from build123d import *

# Parameters (mm, degrees)
SKETCH3_W           = 80
SKETCH3_H           = 110
BOSS_EXTRUDE1_DEPTH = 6
SKETCH4_W           = 6
SKETCH4_H           = 4
BOSS_EXTRUDE2_DEPTH = 6
SKETCH6_W           = 10
SKETCH6_H           = 5
BOSS_EXTRUDE3_DEPTH = 6
SKETCH8_R           = 12.4841
CUT_EXTRUDE1_DEPTH  = 6


with BuildPart() as part:
    # Sketch3 → Boss-Extrude1 (new body)
    with BuildSketch(Plane.XY):
        with Locations((40, 55)):
            Rectangle(SKETCH3_W, SKETCH3_H)
    extrude(amount=BOSS_EXTRUDE1_DEPTH)

    # Sketch4 → Boss-Extrude2 (add)
    with BuildSketch(Plane.XY.offset(6)):
        with Locations((51, -2)):
            Rectangle(SKETCH4_W, SKETCH4_H)
    extrude(amount=-BOSS_EXTRUDE2_DEPTH)

    # Sketch6 → Boss-Extrude3 (add)
    with BuildSketch(Plane.XY.offset(6)):
        with Locations((85, 79.55)):
            Rectangle(SKETCH6_W, SKETCH6_H)
    extrude(amount=-BOSS_EXTRUDE3_DEPTH)

    # Sketch8 → Cut-Extrude1 (cut)
    with BuildSketch(Plane.XY.offset(6)):
        with Locations((27.72, 65.58)):
            Circle(SKETCH8_R)
    extrude(amount=-CUT_EXTRUDE1_DEPTH, mode=Mode.SUBTRACT)


solid = part.part
Work out the finished part from the listing and answer in its coordinate system (mm). A direction names the side the tool comes from. Coordinates: 2 decimals unless noted, no trailing zeros. Order: outer loops, then holes, each group sorted by start corner. A loop starts at its lowest first (then second) coordinate and runs counter-clockwise, first axis right, second up. Notation, with made-up numbers: (-31.5, 81) - (-16.5, 81) arc R31 cw to (-16.5, 112) - close; hole circle Ø4 at (-22, 37). An arc over 180 degrees is marked (long way). Put each result on its own line as item: value. Start each with the question number.
1) Find the intervals of material crossed by line 1 (X direction, y = 21.5, z = 2.35); line 2 (Y direction, x = 27.72, z = 3.85); line 3 (Y direction, x = 62, z = 3.9), in increasing order. Write a range as from..to.
2) Find section D-D (y = 45.5). Give the vertices of the cut face in (x, z), plus the area to 3 significant figures.
3) Flat-ended cylindrical pins translate along their axes: pin 1 (1.5 mm diameter, centred on x = 10, z = 2, fed in from -Y); pin 2 (2 mm diameter, centred on y = 14.5, z = 0.5, fed in from +X); pin 3 (2 mm diameter, centred on y = -1.5, z = 2.5, fed in from -X). Find the tip coordinate at first contact, or state that the pin passes through.
4) Find section A-A (y = 65.58). Give the vertices of the cut face in (x, z), plus the area to 3 significant figures.
5) For a pull along Y with two mould halves and no side action, classify faces 1 (the flat face through (51, -4, 3)), 2 (the flat face through (44, 54, 6)), 3 (the cylindrical face through (26.095, 77.958, 3.042)) as released by +Y, released by -Y, zero draft, split by the parting line, or undercut.
6) For faces 4 (the flat face through (54, -2, 3)), 5 (the flat face through (80, 96, 3)), 6 (the flat face through (24, 0, 3)), determine the directions among +Z, -Z, +X, -X, +Y, -Y from which every point of the face is accessible in a straight line to the end or side of a thin tool.
7) Find section C-C (x = 10.5). Give the vertices of the cut face in (y, z).
8) Find section B-B (z = 5.1). Give the vertices of the cut face in (x, y).
Results list:
1. line 1: x = 0..80
1. line 2: y = 0..53.1, 78.06..110
1. line 3: y = 0..110
2. outline: (0, 0) - (80, 0) - (80, 6) - (0, 6) - close
2. area: 480 mm^2
3. pin 1: stops at y = 0
3. pin 2: stops at x = 80
3. pin 3: stops at x = 48
4. outline: (0, 0) - (15.24, 0) - (15.24, 6) - (0, 6) - close; (40.2, 0) - (80, 0) - (80, 6) - (40.2, 6) - close
4. area: 330 mm^2
5. face 1: released by -Y
5. face 2: zero draft
5. face 3: undercut
6. face 4: +Z, -Z, +X, -Y
6. face 5: +Z, -Z, +X, +Y
6. face 6: +Z, -Z, -X, -Y
7. outline: (0, 0) - (110, 0) - (110, 6) - (0, 6) - close
8. outline: (0, 0) - (48, 0) - (48, -4) - (54, -4) - (54, 0) - (80, 0) - (80, 77.05) - (90, 77.05) - (90, 82.05) - (80, 82.05) - (80, 110) - (0, 110) - close; hole circle Ø24.97 at (27.72, 65.58)
